from build123d import *

# Parameters (mm, degrees)
F0_W     = 500
F0_H     = 500
F1_DEPTH = 3
F3_D     = 15
F5_D     = 12
F7_D     = 12


with BuildPart() as f1:
    # F0 (on Front) → F1 (new body)
    with BuildSketch(Plane.XZ):
        with Locations((250, 250)):
            Rectangle(F0_W, F0_H)
    extrude(amount=F1_DEPTH)

    # F3 (through all)
    with Locations(Plane.XZ.offset(3)):
        with Locations((150, 350), (250, 391.421356), (350, 350), (391.421356, 250), (350, 150), (250, 108.578644), (150, 150), (108.578644, 250)):
            Hole(F3_D / 2)

    # F5 (through all)
    with Locations(Plane.XZ.offset(3)):
        with Locations((25, 325), (25, 475), (175, 475), (325, 475), (475, 475), (475, 325), (475, 175), (475, 25), (325, 25), (175, 25), (25, 25), (25, 175)):
            Hole(F5_D / 2)

    # F7 (through all)
    with Locations(Plane.XZ.offset(3)):
        with Locations((124, 376), (376, 376), (376, 124), (124, 124)):
            Hole(F7_D / 2)


solid = f1.part
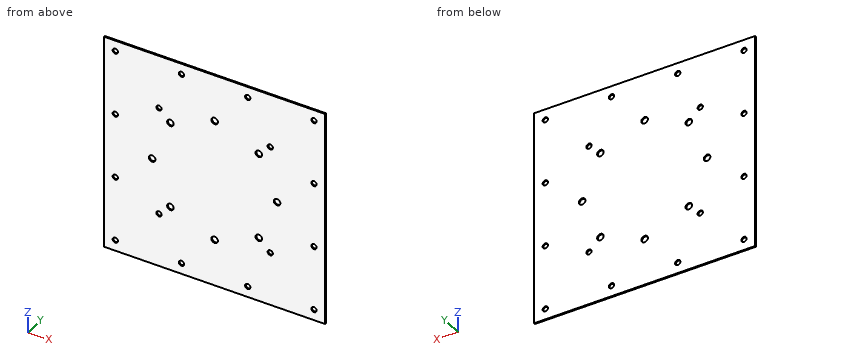
The model under review builds one solid part; all positions refer to its coordinate system, in mm. Coordinates: 2 decimals unless noted, no trailing zeros. Write each loop counter-clockwise with the first axis right and the second up, starting at its lowest first coordinate (ties: lowest second). Pieces come first, ordered by that corner, then holes. Notation, with made-up numbers: M -29,40.5 L -22,40.5 A14 ccw -22,63.5 Z; hole C 64.5,19.5 d10. An arc over 180 degrees is marked long. Put each result on its own line as item: value.
1) Clearance check with a flat-ended pin moving along its axis: pin 1 Ø11 at (x, z) = (475, 475) entering from +Y. State where the tip first meets the part, or that it passes through.
Computed:
pin 1: passes through
2) Add section B-B on x = 475. Give the boundary of the cut face in (y, z), then the cut area to 3 significant figures.
Computed:
outline: M -3,0 L 0,0 L 0,19 L -3,19 Z; M -3,31 L 0,31 L 0,169 L -3,169 Z; M -3,181 L 0,181 L 0,319 L -3,319 Z; M -3,331 L 0,331 L 0,469 L -3,469 Z; M -3,481 L 0,481 L 0,500 L -3,500 Z
area: 1,360 mm2
3) Add section D-D on x = 350. Give the boundary of the cut face in (y, z).
Computed:
outline: M -3,0 L 0,0 L 0,142.5 L -3,142.5 Z; M -3,157.5 L 0,157.5 L 0,342.5 L -3,342.5 Z; M -3,357.5 L 0,357.5 L 0,500 L -3,500 Z
4) Wall thickness on probe 1 along X at (y, z) = (-0.6, 350); probe 2 along X at (y, z) = (-2.2, 376): over which ranges is each line inside the solid? List them lowest first. Write a range as [from, to].
Computed:
probe 1: x = [0, 142.5], [157.5, 342.5], [357.5, 500]
probe 2: x = [0, 118], [130, 370], [382, 500]
5) Add section C-C on z = 124. Give the boundary of the cut face in (x, y).
Computed:
outline: M 0,-3 L 118,-3 L 118,0 L 0,0 Z; M 130,-3 L 370,-3 L 370,0 L 130,0 Z; M 382,-3 L 500,-3 L 500,0 L 382,0 Z
6) Add section A-A on z = 475. Give the boundary of the cut face in (x, y), then the cut area to 3 significant figures.
Computed:
outline: M 0,-3 L 19,-3 L 19,0 L 0,0 Z; M 31,-3 L 169,-3 L 169,0 L 31,0 Z; M 181,-3 L 319,-3 L 319,0 L 181,0 Z; M 331,-3 L 469,-3 L 469,0 L 331,0 Z; M 481,-3 L 500,-3 L 500,0 L 481,0 Z
area: 1,360 mm2
